Drawing for the job (mm, zero at the part's lowest x, y, z). A direction names the side the tool comes from. Coordinates: 2 decimals unless noted, no trailing zeros. Write each loop counter-clockwise with the first axis right and the second up, starting at its lowest first coordinate (ties: lowest second). Pieces come first, ordered by that corner, then holes. Notation, with made-up numbers: (43, -36.5) -> (64, -36.5) arc R12 ccw to (64, -13.5) -> close; hole circle Ø1 at (-24.75, 58). An arc over 180 degrees is marked (long way). Write each question's results on one line, items separated by ' | '. Start each with the question number.
Q1. Saw through at A-A on z = 5. Give the cut face in (x, y).
Q2. Drop flat-ended pins along their axis: pin 1 Ø3.5 at (x, z) = (4.5, 4.5) entering from +Y; pin 2 Ø3 at (x, z) = (9.5, 10.5) entering from -Y; pin 3 Ø5 at (x, y) = (5, 41) entering from -Z; pin 4 Ø3 at (x, z) = (5, 5) entering from -Y. Give the stop position or say it passes through.
Q3. Saw through at D-D on y = 5. Give the cut face in (x, z), and give its area (3 significant figures).
Q4. Drill centre lines: line 1 (Y direction, x = 5, z = 17); line 2 (X direction, y = 1.9, z = 15); line 3 (Y direction, x = 6, z = 20.25). Where is each one in solid material? Low to high.
Q5. Two-plate mould, pull along Y, no slides. Class the marked faces 4, 5 and 6: released by +Y, released by -Y, zero draft, split by the parting line, or undercut.
Q6. Saw through at C-C on z = 15.75. Give the cut face in (x, y).
Q7. Tool access for the marked faces 1, 2 and 3: list every direction of +Z, -Z, +X, -X, +Y, -Y with a clear straight run to the whole face (end or side of a thin tool).
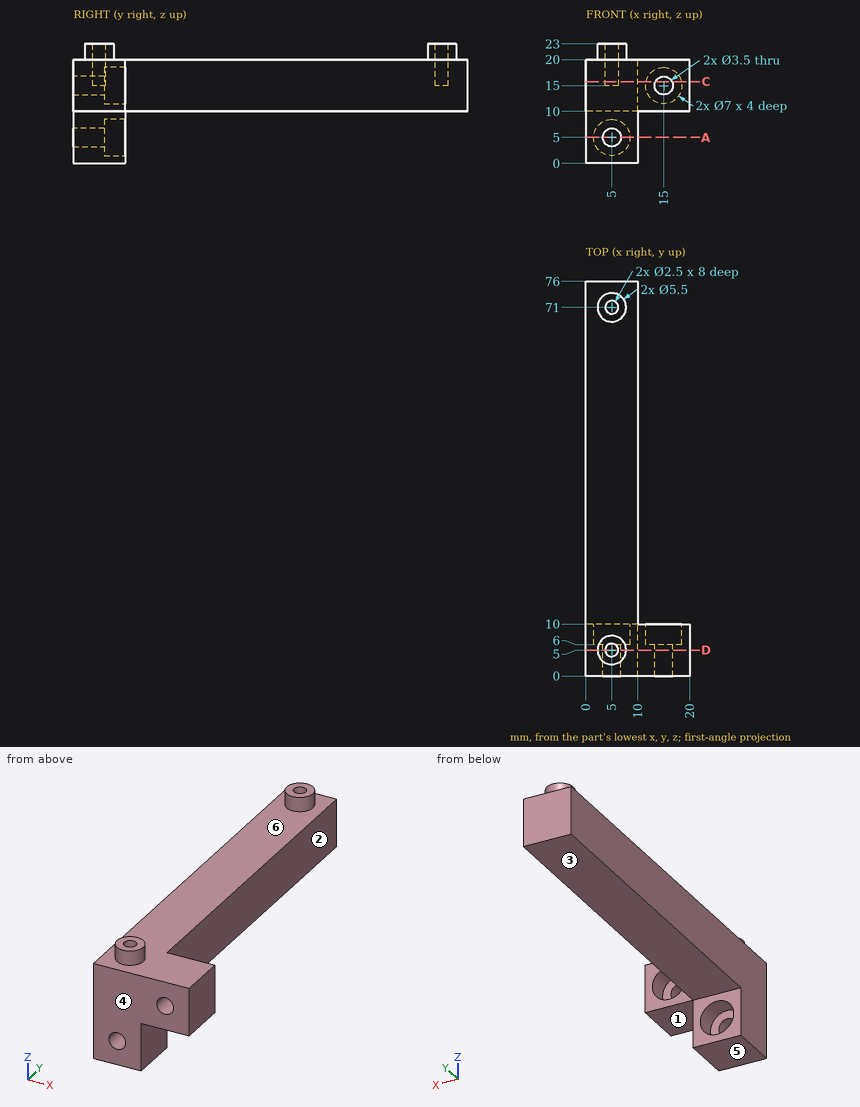
Returned:
1) outline: (0, 0) -> (3.25, 0) -> (3.25, 6) -> (1.5, 6) -> (1.5, 10) -> (0, 10) -> close; (6.75, 0) -> (10, 0) -> (10, 10) -> (8.5, 10) -> (8.5, 6) -> (6.75, 6) -> close
2) pin 1: stops at y = 6 | pin 2: stops at y = 0 | pin 3: stops at z = 10 | pin 4: passes through
3) outline: (0, 0) -> (10, 0) -> (10, 10) -> (20, 10) -> (20, 20) -> (7.75, 20) -> (7.75, 23) -> (6.25, 23) -> (6.25, 15) -> (3.75, 15) -> (3.75, 23) -> (2.25, 23) -> (2.25, 20) -> (0, 20) -> close; hole circle Ø3.5 at (5, 5); hole circle Ø3.5 at (15, 15) | area: 277 mm2
4) line 1: y = 0 to 3.75, 6.25 to 69.75, 72.25 to 76 | line 2: x = 0 to 13.25, 16.75 to 20 | line 3: y = 2.44 to 4.25, 5.75 to 7.56, 68.44 to 70.25, 71.75 to 73.56
5) face 4: released by -Y | face 5: zero draft | face 6: undercut
6) outline: (0, 0) -> (13.42, 0) -> (13.42, 6) -> (11.58, 6) -> (11.58, 10) -> (10, 10) -> (10, 76) -> (0, 76) -> close; (16.58, 0) -> (20, 0) -> (20, 10) -> (18.42, 10) -> (18.42, 6) -> (16.58, 6) -> close; hole circle Ø2.5 at (5, 5); hole circle Ø2.5 at (5, 71)
7) face 1: -Z, +X, +Y, -Y | face 2: +Z, -Z, +X, +Y | face 3: -Z, +X, -X, +Y
